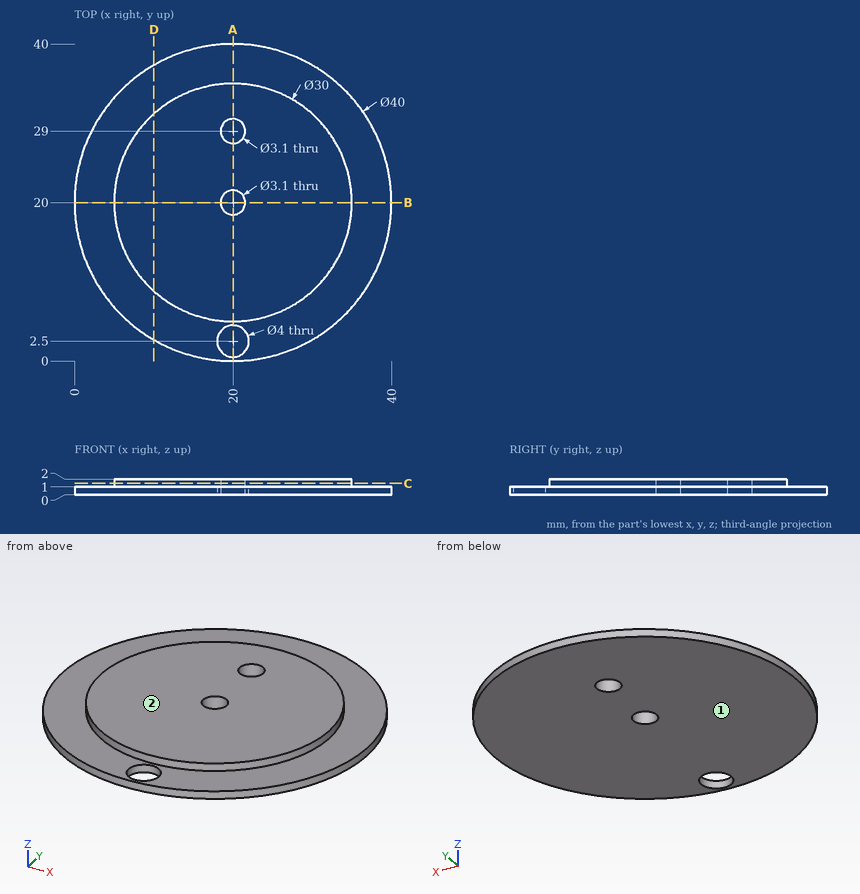
Print and shaded views of the part. All mm, measured from the part's lowest x, y and z. Coordinates: 2 decimals unless noted, no trailing zeros. Write each loop counter-clockwise with the first axis right and the second up, starting at its lowest first coordinate (ties: lowest second). Pieces come first, ordered by that corner, then holes.
(1) Drill centre lines: probe 1 along Y at (x, z) = (20, 0.7); probe 2 along Y at (x, z) = (20, 1.35); probe 3 along Z at (x, y) = (6.5, 28.5). Where is each one in solid material? Low to high.
(2) Cut at B-B, the plane y = 20. List the corners of the cut face in (x, z).
(3) Cut at C-C, the plane z = 1.45. List the corners of the cut face in (x, y), and give its area (3 significant figures).
(4) Two-plate mould, pull along Z, no slides. Class the marked faces 1 and 2: +Z half, -Z half, draft (parallel to the pull), parting line (faces both ways), or undercut.
(5) Cut at A-A, the plane x = 20. List the corners of the cut face in (y, z).
(6) Flat gauge pins, fed straight in: pin 1 (1 mm diameter, centred on x = 7, y = 29.5, fed in from +Z); pin 2 (1.9 mm diameter, centred on x = 20, y = 20, fed in from +Z). Where does each tip first touch, or does it go through?
(7) Cut at D-D, the plane x = 10. List the corners of the cut face in (y, z).
Geometry says:
1. probe 1: y = 0 to 0.5, 4.5 to 18.45, 21.55 to 27.45, 30.55 to 40
1. probe 2: y = 5 to 18.45, 21.55 to 27.45, 30.55 to 35
1. probe 3: z = 0 to 1
2. outline: (0, 0) - (18.45, 0) - (18.45, 2) - (5, 2) - (5, 1) - (0, 1) - close; (21.55, 0) - (40, 0) - (40, 1) - (35, 1) - (35, 2) - (21.55, 2) - close
3. outline: circle Ø30 at (20, 20); hole circle Ø3.1 at (20, 20); hole circle Ø3.1 at (20, 29)
3. area: 692 mm2
4. face 1: -Z half
4. face 2: +Z half
5. outline: (0, 0) - (0.5, 0) - (0.5, 1) - (0, 1) - close; (4.5, 0) - (18.45, 0) - (18.45, 2) - (5, 2) - (5, 1) - (4.5, 1) - close; (21.55, 0) - (27.45, 0) - (27.45, 2) - (21.55, 2) - close; (30.55, 0) - (40, 0) - (40, 1) - (35, 1) - (35, 2) - (30.55, 2) - close
6. pin 1: stops at z = 1
6. pin 2: passes through
7. outline: (2.68, 0) - (37.32, 0) - (37.32, 1) - (31.18, 1) - (31.18, 2) - (8.82, 2) - (8.82, 1) - (2.68, 1) - close
